```python
from build123d import *

# Parameters (mm, degrees)
BOSS_EXTRUDE1_DEPTH = 15
SKETCH2_R           = 4
CUT_EXTRUDE1_DEPTH  = 64.763255305
FILLET1_R           = 3
SKETCH4_R           = 5
BOSS_EXTRUDE2_DEPTH = 15
SKETCH5_R           = 3
CUT_EXTRUDE2_DEPTH  = 7


with BuildPart() as part:
    # Sketch1 → Boss-Extrude1 (new body)
    with BuildSketch(Plane.XY):
        Polygon((0, 0), (42, 0), (42, -55.763255305), (0, -55.763255305), (0, -59.763255305), (46, -59.763255305), (46, 4), (0, 4), align=None)
    extrude(amount=BOSS_EXTRUDE1_DEPTH)

    # Sketch2 → Cut-Extrude1 (cut, through all)
    with BuildSketch(Plane(origin=(0, 4, 0), x_dir=(1, 0, 0), z_dir=(0, 1, 0))):
        with Locations((8, -7.5)):
            Circle(SKETCH2_R)
    extrude(amount=-CUT_EXTRUDE1_DEPTH, mode=Mode.SUBTRACT)

    # Fillet1
    fillet1_edges = [part.edges().sort_by_distance(p)[0] for p in [
        (46, 4, 7.5),
        (46, -59.763255305, 7.5),
        (42, -55.763255305, 7.5),
        (42, 0, 7.5),
    ]]
    fillet(fillet1_edges, radius=FILLET1_R)

    # Sketch4 → Boss-Extrude2 (add)
    with BuildSketch(Plane(origin=(46, 0, 0), x_dir=(0, 0, -1), z_dir=(1, 0, 0))):
        with Locations((-7.5, -27.881627652)):
            Circle(SKETCH4_R)
    extrude(amount=BOSS_EXTRUDE2_DEPTH)

    # Sketch5 → Cut-Extrude2 (cut)
    with BuildSketch(Plane.XY):
        with Locations((56, -27.881627652)):
            Circle(SKETCH5_R)
    extrude(amount=CUT_EXTRUDE2_DEPTH, mode=Mode.SUBTRACT)


solid = part.part
```
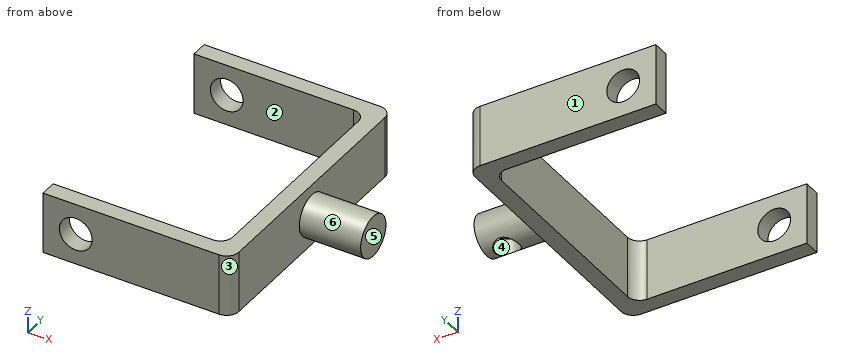
Design review of the part built by this model. Coordinates are the model's own, in mm. Face numbers are marked on the shaded views. A direction names the side the tool comes from. Give positions to 0.01 mm unless a question says otherwise; leave off trailing zeros. Order: outer loops, then holes, each group sorted by start corner. A loop starts at its lowest first (then second) coordinate and runs counter-clockwise, first axis right, second up. Notation, with made-up numbers: (-39.5, -15.75) -> (9.5, -15.75) arc R28 ccw to (9.5, 11.25) -> close; hole circle Ø11 at (-1, -2). An arc over 180 degrees is marked (long way). Write each question's results on one line, items separated by ' | '. Start each with the question number.
Q1. Add section B-B on z = 5.75. Give the boundary of the cut face in (x, y), and give its area (3 significant figures).
Q2. Add section D-D on z = 9.5. Give the boundary of the cut face in (x, y), and give its area (3 significant figures).
Q3. Add section C-C on z = 1.75. Give the boundary of the cut face in (x, y).
Q4. For pin 1 (7 mm diameter, centred on x = 56, y = -27.88, fed in from +Z); pin 2 (1.5 mm diameter, centred on x = 54.5, z = 7.5, fed in from +Y); pin 3 (4 mm diameter, centred on y = -44, z = 4.5, fed in from +X), all flat-tipped, find the tip position at first contact; note any pin that passes through.
Q5. Machinability: for the marked faces 1 and 2, which of the approach directions +Z, -Z, +X, -X, +Y, -Y give a long, thin tool a straight path to every point of the face, cutting with its end or side? Answer none if there is none.
Q6. Mouldability with a two-part tool opening along Y and no side actions: class the marked faces 3, 4, 5 and 6 as +Y half, -Y half, draft (parallel to the pull), parting line (faces both ways), or undercut.
Q7. Add section A-A on x = 13. Give the boundary of the cut face in (y, z).
Q8. Wall thickness on L1, parallel to Y at x = 22, z = 12; L2, parallel to X at y = -40.5, z = 5; L3, parallel to Y at x = 40.5, z = 8.75: over which ranges is each line inside the solid? List them lowest first. Write a range as from..to.
Found:
1) outline: (0, -59.76) -> (4.4, -59.76) -> (4.4, -55.76) -> (0, -55.76) -> close; (0, 0) -> (4.4, 0) -> (4.4, 4) -> (0, 4) -> close; (11.6, -59.76) -> (43, -59.76) arc R3 ccw to (46, -56.76) -> (46, -32.57) -> (61, -32.57) -> (61, -23.2) -> (46, -23.2) -> (46, 1) arc R3 ccw to (43, 4) -> (11.6, 4) -> (11.6, 0) -> (39, 0) arc R3 cw to (42, -3) -> (42, -52.76) arc R3 cw to (39, -55.76) -> (11.6, -55.76) -> close; hole circle Ø6 at (56, -27.88) | area: 646 mm2
2) outline: (0, -59.76) -> (4.54, -59.76) -> (4.54, -55.76) -> (0, -55.76) -> close; (0, 0) -> (4.54, 0) -> (4.54, 4) -> (0, 4) -> close; (11.46, -59.76) -> (43, -59.76) arc R3 ccw to (46, -56.76) -> (46, -32.46) -> (61, -32.46) -> (61, -23.3) -> (46, -23.3) -> (46, 1) arc R3 ccw to (43, 4) -> (11.46, 4) -> (11.46, 0) -> (39, 0) arc R3 cw to (42, -3) -> (42, -52.76) arc R3 cw to (39, -55.76) -> (11.46, -55.76) -> close | area: 673 mm2
3) outline: (0, -59.76) -> (43, -59.76) arc R3 ccw to (46, -56.76) -> (46, 1) arc R3 ccw to (43, 4) -> (0, 4) -> (0, 0) -> (39, 0) arc R3 cw to (42, -3) -> (42, -52.76) arc R3 cw to (39, -55.76) -> (0, -55.76) -> close
4) pin 1: stops at z = 12.5 | pin 2: stops at y = -22.88 | pin 3: stops at x = 46
5) face 1: +Z, -Z, +X, -X, +Y | face 2: +Z, -Z, -X
6) face 3: -Y half | face 4: undercut | face 5: draft | face 6: parting line
7) outline: (-59.76, 0) -> (-55.76, 0) -> (-55.76, 15) -> (-59.76, 15) -> close; (0, 0) -> (4, 0) -> (4, 15) -> (0, 15) -> close
8) L1: y = -59.76..-55.76, 0..4 | L2: x = 42..46 | L3: y = -59.76..-55.36, -0.4..4
